For this review, take the finished solid that the model builds, in its own axes (mm). A direction names the side the tool comes from. Give positions to 0.01 mm unless a question says otherwise; leave off trailing zeros. Loops run counter-clockwise (first coordinate to the right, second up) from the corner with the lowest first, then second, coordinate; pieces in that order, holes last. Notation, with made-up numbers: (33, -10.5) - (57, -10.5) arc R4 cw to (57, -6.5) - close; hole circle Ø3 at (-3.5, -13.75). An arc over 180 degrees is marked (long way). Put each result on its own line as item: value. Start each with the question number.
from build123d import *

# Parameters (mm, degrees)
F1_DEPTH = 10
F2_R     = 4.1
F3_DEPTH = 5
F4_DEPTH = 10
F5_R     = 1
F6_R     = 4.99999
F7_R     = 5


# Not quite as in the source:
# - a fillet or chamfer is up to 0.001 mm smaller than in the source, because OpenCascade refuses the exact size


with BuildPart() as f1:
    # F0 (on Top) → F1 (new body)
    with BuildSketch(Plane.XY):
        with BuildLine():
            Line((23.4835705605, 25.9523007406), (0, 0))
            Line((0, 0), (-43.0009548823, 0))
            ThreePointArc((-43.0009548823, 0), (-49.0004774411, -5.9243094089), (-55, 0))
            Line((-55, 0), (-60, 0))
            Line((-60, 0), (-60, -10))
            Line((-60, -10), (17.0862320811, -10))
            Line((17.0862320811, -10), (40.5698026416, 15.9523007406))
            Line((40.5698026416, 15.9523007406), (98.4835705605, 15.9523007406))
            Line((98.4835705605, 15.9523007406), (98.4835705605, 25.9523007406))
            Line((98.4835705605, 25.9523007406), (23.4835705605, 25.9523007406))
        make_face()
    extrude(amount=F1_DEPTH)

    # F2 (on face) → F3 (cut)
    with BuildSketch(Plane.XY.offset(10)):
        Polygon((0, -10), (17.0862320811, -10), (40.5698026416, 15.9523007406), (40.5698026416, 25.9523007406), (23.4835705605, 25.9523007406), (0, 0), align=None)
        with Locations((12.5, 0.5)):
            Circle(F2_R, mode=Mode.SUBTRACT)
    extrude(amount=-F3_DEPTH, mode=Mode.SUBTRACT)

    # F4 (cut, through all): a face of the model
    f4_faces = [f1.faces().sort_by_distance(p)[0] for p in [
        (12.5, 0.5, 10),
    ]]
    extrude(f4_faces, amount=-F4_DEPTH, mode=Mode.SUBTRACT)

    # F5
    f5_edges = [f1.edges().sort_by_distance(p)[0] for p in [
        (60.983571, 25.952301, 0),
        (69.526687, 25.952301, 10),
        (98.483571, 25.952301, 5),
        (98.483571, 20.952301, 0),
        (98.483571, 20.952301, 10),
        (98.483571, 15.952301, 5),
        (69.526687, 15.952301, 0),
        (69.526687, 15.952301, 10),
        (23.483571, 25.952301, 2.5),
        (17.086232, -10, 2.5),
        (40.569803, 15.952301, 2.5),
        (28.828017, 2.97615, 0),
    ]]
    fillet(f5_edges, radius=F5_R)

    # F6 (radius 5 in the source; OpenCascade refuses exactly that, so slightly less here)
    f6_edges = [f1.edges().sort_by_distance(p)[0] for p in [
        (40.569803, 20.952301, 5),
    ]]
    fillet(f6_edges, radius=F6_R)

    # F7
    f7_edges = [f1.edges().sort_by_distance(p)[0] for p in [
        (0, 0, 7.5),
    ]]
    fillet(f7_edges, radius=F7_R)


solid = f1.part
1) Insertion check: P1, Ø1.5, axis at y = -7, z = 6.5, coming from the +X side; P2, Ø5, axis at x = -29, z = 5.5, coming from the +Y side; P3, Ø5, axis at x = 50, z = 7.5, coming from the -Y side. Each pin has a flat end and moves straight along its axis. Give the tip position at first contact, or say it passes through.
2) Mouldability with a two-part tool opening along Y and no side actions: class faces 4 (the cylindrical face through (8.404, 0.68, 2.535)), 5 (the cylindrical face through (-1, -2, 8)), 6 (the flat face through (66, 15.952, 5)) as released by +Y, released by -Y, zero draft, split by the parting line, or undercut.
3) Take a section at A-A on z = 6.75. State the section outline as (x, y) points.
4) Take a section at D-D on x = 66. State the section outline as (y, z) points, and give its area (3 significant figures).
5) Wall thickness on probe 1 along Y at (x, z) = (79, 2.25); probe 2 along X at (y, z) = (-3.5, 7.5); probe 3 along Z at (x, y) = (33, 16): over which ranges is each line inside the solid? List them lowest first.
6) Take a section at B-B on x = 12.5. State the section outline as (y, z) points.
7) Machinability: for faces 1 (the flat face through (28.67, 2.8, 2.97)), 2 (the flat face through (-57, 0, 5)), 3 (the flat face through (0, -7, 8)), which of the approach directions +Z, -Z, +X, -X, +Y, -Y give a long, thin tool a straight path to every point of the face, cutting with its end or side? Answer none if there is none.
Answers follow:
1. P1: x = 0
1. P2: y = 0
1. P3: y = 15.95
2. face 4: undercut
2. face 5: released by +Y
2. face 6: released by -Y
3. outline: (-60, -10) - (0, -10) - (0, -5) arc R5 ccw to (-5, 0) - (-43, 0) arc R6 cw to (-55, 0) - (-60, 0) - close; (39.37, 15.95) - (97.48, 15.95) arc R1 ccw to (98.48, 16.95) - (98.48, 24.95) arc R1 ccw to (97.48, 25.95) - (39.37, 25.95) - close
4. outline: (15.95, 1) arc R1 ccw to (16.95, 0) - (24.95, 0) arc R1 ccw to (25.95, 1) - (25.95, 9) arc R1 ccw to (24.95, 10) - (16.95, 10) arc R1 ccw to (15.95, 9) - close
4. area: 99.1 mm2
5. probe 1: 15.95 to 25.95
5. probe 2: -60 to -53.82, -44.18 to -0.23
5. probe 3: 0 to 5
6. outline: (-10, 0) - (-3.6, 0) - (-3.6, 5) - (-10, 5) - close; (4.6, 0) - (13.81, 0) - (13.81, 5) - (4.6, 5) - close
7. face 1: +Z, -Z, +X, -Y
7. face 2: +Z, -Z, -X, +Y
7. face 3: +Z, +X, +Y, -Y
